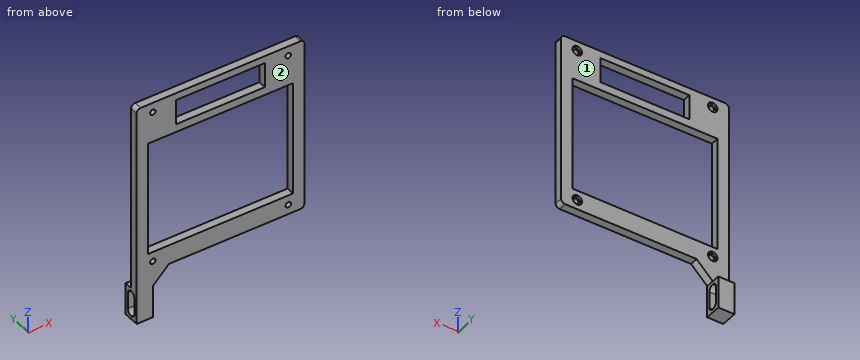
from build123d import *

# Parameters (mm, degrees)
SKETCH1_W                                      = 132.08
SKETCH1_H                                      = 137.16
BOSS_EXTRUDE1_DEPTH                            = 6.35
CBORE_FOR_6_BUTTON_HEAD_CAP_SCREW1_D           = 4.3053
CBORE_FOR_6_BUTTON_HEAD_CAP_SCREW1_CBORE_D     = 7.54126
CBORE_FOR_6_BUTTON_HEAD_CAP_SCREW1_CBORE_DEPTH = 1.8542
SKETCH5_W                                      = 114.3
SKETCH5_H                                      = 106.68
CUT_EXTRUDE1_DEPTH                             = 191.521165491
SKETCH6_W                                      = 12.7
SKETCH6_H                                      = 38.1
BOSS_EXTRUDE2_DEPTH                            = 6.35
SKETCH7_W                                      = 12.7
SKETCH7_H                                      = 6.35
BOSS_EXTRUDE3_DEPTH                            = 25.4
CUT_EXTRUDE2_REACH                             = 221.824
CHAMFER1_SIZE                                  = 12.7
CUT_EXTRUDE3_REACH                             = 221.548
SKETCH9_W                                      = 69.85
SKETCH9_H                                      = 9.525
FILLET1_R                                      = 3.175
BOSS_EXTRUDE4_DEPTH                            = 6.35


with BuildPart() as part:
    # Sketch1 → Boss-Extrude1 (new body)
    with BuildSketch(Plane(origin=(0, 0, 0), x_dir=(1, 0, 0), z_dir=(0, 1, 0))):
        with Locations((66.04, 68.58)):
            Rectangle(SKETCH1_W, SKETCH1_H)
    extrude(amount=BOSS_EXTRUDE1_DEPTH)

    # CBORE for #6 Button Head Cap Screw1 (through all)
    with Locations(Plane(origin=(0, 6.35, 0), x_dir=(1, 0, 0), z_dir=(0, 1, 0))):
        with Locations((12.7, 129.54), (119.38, 129.54), (119.38, 7.62), (12.7, 7.62)):
            CounterBoreHole(CBORE_FOR_6_BUTTON_HEAD_CAP_SCREW1_D / 2, CBORE_FOR_6_BUTTON_HEAD_CAP_SCREW1_CBORE_D / 2, CBORE_FOR_6_BUTTON_HEAD_CAP_SCREW1_CBORE_DEPTH)

    # Sketch5 → Cut-Extrude1 (cut, through all)
    with BuildSketch(Plane(origin=(0, 6.35, 0), x_dir=(1, 0, 0), z_dir=(0, 1, 0))):
        with Locations((66.04, 68.58)):
            Rectangle(SKETCH5_W, SKETCH5_H)
    extrude(amount=-CUT_EXTRUDE1_DEPTH, mode=Mode.SUBTRACT)

    # Sketch6 → Boss-Extrude2 (add)
    with BuildSketch(Plane(origin=(0, 0, 0), x_dir=(-1, 0, 0), z_dir=(0, -1, 0))):
        with Locations((-6.35, 156.21)):
            Rectangle(SKETCH6_W, SKETCH6_H)
    extrude(amount=-BOSS_EXTRUDE2_DEPTH)

    # Sketch7 → Boss-Extrude3 (add)
    with BuildSketch(Plane(origin=(0, 0, -175.26), x_dir=(-1, 0, 0), z_dir=(0, 0, -1))):
        with Locations((-6.35, 9.525)):
            Rectangle(SKETCH7_W, SKETCH7_H)
    extrude(amount=-BOSS_EXTRUDE3_DEPTH)

    # Sketch8 → Cut-Extrude2 (cut, up to next)
    with BuildSketch(Plane.ZY, mode=Mode.PRIVATE) as cut_extrude2_sk1:
        with BuildLine():
            Line((-152.4, 6.35), (-172.72, 6.35))
            ThreePointArc((-172.72, 6.35), (-171.604076836, 3.655923164), (-168.91, 2.54))
            Line((-168.91, 2.54), (-156.21, 2.54))
            ThreePointArc((-156.21, 2.54), (-153.515923164, 3.655923164), (-152.4, 6.35))
        make_face()
    cut_extrude2_tool1 = extrude(cut_extrude2_sk1.sketch, amount=-CUT_EXTRUDE2_REACH, mode=Mode.PRIVATE) & part.part
    # Sketch8 → Cut-Extrude2 (cut, up to next)
    with BuildSketch(Plane.ZY, mode=Mode.PRIVATE) as cut_extrude2_sk2:
        with BuildLine():
            ThreePointArc((-168.91, 10.16), (-171.604076836, 9.044076836), (-172.72, 6.35))
            Line((-172.72, 6.35), (-152.4, 6.35))
            ThreePointArc((-152.4, 6.35), (-153.515923164, 9.044076836), (-156.21, 10.16))
            Line((-156.21, 10.16), (-168.91, 10.16))
        make_face()
    cut_extrude2_tool2 = extrude(cut_extrude2_sk2.sketch, amount=-CUT_EXTRUDE2_REACH, mode=Mode.PRIVATE) & part.part
    add(cut_extrude2_tool1.solids().sort_by_distance((0, 4.537242, -162.56))[0], mode=Mode.SUBTRACT)
    add(cut_extrude2_tool2.solids().sort_by_distance((0, 8.162758, -162.56))[0], mode=Mode.SUBTRACT)

    # Chamfer1
    chamfer1_edges = [part.edges().sort_by_distance(p)[0] for p in [
        (12.7, 3.175, -137.16),
    ]]
    chamfer(chamfer1_edges, length=CHAMFER1_SIZE)

    # Sketch9 → Cut-Extrude3 (cut, up to next)
    with BuildSketch(Plane(origin=(0, 6.35, 0), x_dir=(1, 0, 0), z_dir=(0, 1, 0)), mode=Mode.PRIVATE) as cut_extrude3_sk1:
        with Locations((66.04, 10.4775)):
            Rectangle(SKETCH9_W, SKETCH9_H)
    cut_extrude3_tool1 = extrude(cut_extrude3_sk1.sketch, amount=-CUT_EXTRUDE3_REACH, mode=Mode.PRIVATE) & part.part
    add(cut_extrude3_tool1.solids().sort_by_distance((66.04, 6.35, -10.4775))[0], mode=Mode.SUBTRACT)

    # Fillet1
    fillet1_edges = [part.edges().sort_by_distance(p)[0] for p in [
        (132.08, 3.175, -137.16),
        (132.08, 3.175, 0),
        (0, 3.175, 0),
    ]]
    fillet(fillet1_edges, radius=FILLET1_R)

    # Sketch11 → Boss-Extrude4 (add)
    with BuildSketch(Plane(origin=(0, 6.35, 0), x_dir=(1, 0, 0), z_dir=(0, 1, 0))):
        Polygon((8.89, 15.24), (31.115, 15.24), (31.115, 25.4), (100.965, 25.4), (100.965, 15.24), (123.19, 15.24), (123.19, 31.75), (8.89, 31.75), align=None)
    extrude(amount=-BOSS_EXTRUDE4_DEPTH)


solid = part.part
Part model, mm, in its own coordinate system. Face numbers are marked on the shaded views. A direction names the side the tool comes from. Round coordinates to 2 decimals unless told otherwise and drop trailing zeros. Write each loop counter-clockwise with the first axis right and the second up, starting at its lowest first coordinate (ties: lowest second). Pieces come first, ordered by that corner, then holes. Notation, with made-up numbers: (-25.75, 24) - (13.25, 24) arc R21 cw to (13.25, 53) - close; hole circle Ø3 at (65.25, 27.25). An arc over 180 degrees is marked (long way). Use CSV: the item, a comma, the result in double quotes.
Item 1: Wall check: L1, parallel to Z at x = 51.5, y = 2.5 (3 decimals); L2, parallel to Z at x = 119.38, y = 5.4; L3, parallel to Z at x = 119.38, y = 1.45. Give the ranges that are in metal, low to high.
Results list:
L1,"z = -137.16 to -121.92, -31.75 to -25.4, -5.715 to 0"
L2,"z = -137.16 to -133.31, -125.77 to -121.92, -31.75 to -11.39, -3.85 to 0"
L3,"z = -137.16 to -131.69, -127.39 to -121.92, -31.75 to -9.77, -5.47 to 0"
Item 2: Slice it at D-D, the plane x = 70. Write the cut outline in (y, z) (3 decimals).
Results list:
outline,"(0, -137.16) - (6.35, -137.16) - (6.35, -121.92) - (0, -121.92) - close; (0, -31.75) - (6.35, -31.75) - (6.35, -25.4) - (0, -25.4) - close; (0, -5.715) - (6.35, -5.715) - (6.35, 0) - (0, 0) - close"
Item 3: Slice it at C-C, the plane z = -48.5. Write the cut outline in (x, y), then the cut area to 3 significant figures.
Results list:
outline,"(0, 0) - (8.89, 0) - (8.89, 6.35) - (0, 6.35) - close; (123.19, 0) - (132.08, 0) - (132.08, 6.35) - (123.19, 6.35) - close"
area,"113 mm²"
Item 4: Slice it at A-A, the plane z = -7.62. Write the cut outline in (x, y) (3 decimals).
Results list:
outline,"(0, 0) - (10.547, 0) - (10.547, 4.496) - (8.929, 4.496) - (8.929, 6.35) - (0, 6.35) - close; (14.853, 0) - (31.115, 0) - (31.115, 6.35) - (16.471, 6.35) - (16.471, 4.496) - (14.853, 4.496) - close; (100.965, 0) - (117.227, 0) - (117.227, 4.496) - (115.609, 4.496) - (115.609, 6.35) - (100.965, 6.35) - close; (121.533, 0) - (132.08, 0) - (132.08, 6.35) - (123.151, 6.35) - (123.151, 4.496) - (121.533, 4.496) - close"
Item 5: Slice it at B-B, the plane x = 119.38. Write the cut outline in (y, z), then the cut area to 3 significant figures.
Results list:
outline,"(0, -137.16) - (6.35, -137.16) - (6.35, -133.31) - (4.5, -133.31) - (4.5, -131.69) - (0, -131.69) - close; (0, -127.39) - (4.5, -127.39) - (4.5, -125.77) - (6.35, -125.77) - (6.35, -121.92) - (0, -121.92) - close; (0, -31.75) - (6.35, -31.75) - (6.35, -11.39) - (4.5, -11.39) - (4.5, -9.77) - (0, -9.77) - close; (0, -5.47) - (4.5, -5.47) - (4.5, -3.85) - (6.35, -3.85) - (6.35, 0) - (0, 0) - close"
area,"232 mm²"
Item 6: Tool access for the marked faces 1 and 2: list every direction of +Z, -Z, +X, -X, +Y, -Y with a clear straight run to the whole face (end or side of a thin tool).
Results list:
face 1,"+Z, +X, -X, +Y"
face 2,"+Z, -Z, +X, -X, -Y"
Item 7: Flat gauge pins, fed straight in: P1, Ø5, axis at x = 87, y = 4, coming from the -Z side; P2, Ø6, axis at y = 3.5, z = -141.5, coming from the +X side; P3, Ø8.5, axis at x = 11.5, z = -128.5, coming from the +Y side; P4, Ø4, axis at x = 12.7, z = -129.54, coming from the -Y side. Where does each tip first touch, or does it go through?
Results list:
P1,"stops at z = -137.16"
P2,"stops at x = 24.06"
P3,"stops at y = 6.35"
P4,"passes through"
